```python
from build123d import *

# Parameters (mm, degrees)
F0_R          = 20
F1_DEPTH      = 2.5
F2_R          = 2.5
F3_DEPTH      = 42.5
F4_W          = 42.362636
F4_H          = 7.5
F5_DEPTH      = 5
F6_R          = 2.5
F7_R          = 3.75
F8_DEPTH      = 19.6
F8_DEPTH_BACK = 19.6


with BuildPart() as f1:
    # F0 (on Front) → F1 (new body, symmetric)
    with BuildSketch(Plane.XZ):
        Circle(F0_R)
    extrude(amount=F1_DEPTH, both=True)

    # F2 (on Top) → F3 (join)
    with BuildSketch(Plane.XY):
        Circle(F2_R)
    extrude(amount=F3_DEPTH)

    # F4 (on face) → F5 (join)
    with BuildSketch(Plane.XY.offset(42.5)):
        Rectangle(F4_W, F4_H)
        with BuildLine():
            ThreePointArc((21.181318, -3.75), (24.931318, 0), (21.181318, 3.75))
            Line((21.181318, 3.75), (21.181318, -3.75))
        make_face()
    extrude(amount=F5_DEPTH)

    # F6
    f6_edges = [f1.edges().sort_by_distance(p)[0] for p in [
        (0, 3.75, 47.5),
        (0, -3.75, 47.5),
        (24.931318, 0, 47.5),
    ]]
    fillet(f6_edges, radius=F6_R)

    # F7 (on Top) → F8 (join, two sides)
    with BuildSketch(Plane.XY) as f8_sk:
        Circle(F7_R)
    extrude(amount=F8_DEPTH)
    extrude(f8_sk.sketch, amount=-F8_DEPTH_BACK)


solid = f1.part
```
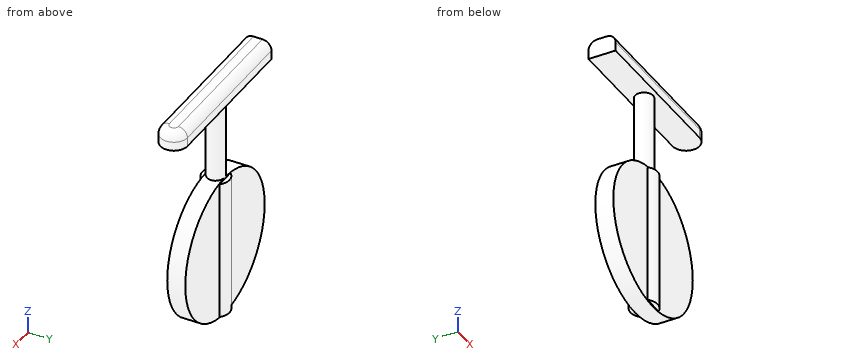
Could you check a few things on this model? Use its own coordinates, in mm. Round coordinates to 2 decimals unless told otherwise and drop trailing zeros. Loops run counter-clockwise (first coordinate to the right, second up) from the corner with the lowest first, then second, coordinate; pieces in that order, holes last. Notation, with made-up numbers: M 28,-31 L 38,-31 A15 ccw 38,-27 Z; hole C 4,13 d8. An arc over 180 degrees is marked long. Put each result on its own line as item: value.
Q1. Imagine slicing it at C-C (x = 1). Write out the boundary of the cut face in (y, z).
Check result:
outline: M -3.75,42.5 L -2.29,42.5 L -2.29,19.97 L -2.5,19.97 L -2.5,19.6 L -3.61,19.6 L -3.61,-19.6 L -2.5,-19.6 L -2.5,-19.97 L 2.5,-19.97 L 2.5,-19.6 L 3.61,-19.6 L 3.61,19.6 L 2.5,19.6 L 2.5,19.97 L 2.29,19.97 L 2.29,42.5 L 3.75,42.5 L 3.75,45 A2.5 ccw 1.25,47.5 L -1.25,47.5 A2.5 ccw -3.75,45 Z
Q2. For pin 1 (6 mm diameter, centred on x = 12, z = -10, fed in from -Y); pin 2 (12 mm diameter, centred on x = -8.5, z = 0.5, fed in from -Y); pin 3 (1.4 mm diameter, centred on x = 0.5, y = -3.5, fed in from -Z); pin 4 (20 mm diameter, centred on x = 2, z = 4.5, fed in from +Y), each with a flat end and sliding along its axis, tell me the tip position at first contact or that it passes through.
Check result:
pin 1: y = -2.5
pin 2: y = -2.8
pin 3: z = -19.6
pin 4: y = 3.75
Q3. Imagine slicing it at A-A (x = 16). Write out the boundary of the cut face in (y, z).
Check result:
outline: M -3.75,42.5 L 3.75,42.5 L 3.75,45 A2.5 ccw 1.25,47.5 L -1.25,47.5 A2.5 ccw -3.75,45 Z; M -2.5,-12 L 2.5,-12 L 2.5,12 L -2.5,12 Z
Q4. I need wall thicknesses on probe 1 along Y at (x, z) = (13, 7); probe 2 along Z at (x, y) = (6.5, -0.5); probe 3 along Z at (x, y) = (22, -1.25). Which ranges of each line are inside material? Lowest first, please.
Check result:
probe 1: -2.5 to 2.5
probe 2: -18.91 to 18.91, 42.5 to 47.5
probe 3: 42.5 to 47.49
Q5. Imagine slicing it at B-B (z = -11.5). Write out the boundary of the cut face in (x, y), then the cut area to 3 significant figures.
Check result:
outline: M -16.36,-2.5 L -2.8,-2.5 A3.75 ccw 2.8,-2.5 L 16.36,-2.5 L 16.36,2.5 L 2.8,2.5 A3.75 ccw -2.8,2.5 L -16.36,2.5 Z
area: 173 mm2
Q6. Imagine slicing it at D-D (z = 4). Write out the boundary of the cut face in (x, y).
Check result:
outline: M -19.6,-2.5 L -2.8,-2.5 A3.75 ccw 2.8,-2.5 L 19.6,-2.5 L 19.6,2.5 L 2.8,2.5 A3.75 ccw -2.8,2.5 L -19.6,2.5 Z
